```python
from build123d import *

# Parameters (mm, degrees)
SKETCH1_W           = 114.3
SKETCH1_H           = 38.1
BOSS_EXTRUDE1_DEPTH = 25.4
CUT_EXTRUDE1_REACH  = 125.131
SKETCH2_W           = 33.528
SKETCH2_H           = 20.828
CUT_EXTRUDE2_REACH  = 125.131
SKETCH3_R           = 1.778
CUT_EXTRUDE3_REACH  = 125.131
SKETCH4_R           = 1.778
CUT_EXTRUDE4_REACH  = 125.131
SKETCH5_R           = 1.778
SKETCH5_R_2         = 6.35
CUT_EXTRUDE5_REACH  = 125.131
SKETCH6_R           = 1.778
SKETCH6_R_2         = 6.35
CUT_EXTRUDE6_REACH  = 125.131
SKETCH7_R           = 1.778
SKETCH7_R_2         = 6.35
CUT_EXTRUDE7_REACH  = 125.131
SKETCH8_R           = 1.778
SKETCH8_R_2         = 6.35
CUT_EXTRUDE8_REACH  = 125.131
SKETCH9_R           = 1.778
CUT_EXTRUDE9_REACH  = 125.131
SKETCH10_R          = 1.778


with BuildPart() as part:
    # Sketch1 → Boss-Extrude1 (new body)
    with BuildSketch(Plane(origin=(0, 0, 0), x_dir=(1, 0, 0), z_dir=(0, 1, 0))):
        with Locations((-57.15, -19.05)):
            Rectangle(SKETCH1_W, SKETCH1_H)
    extrude(amount=BOSS_EXTRUDE1_DEPTH)

    # Sketch2 → Cut-Extrude1 (cut, up to next)
    with BuildSketch(Plane(origin=(0, 0, 0), x_dir=(0, 0, -1), z_dir=(1, 0, 0)), mode=Mode.PRIVATE) as cut_extrude1_sk1:
        with Locations((-19.05, 12.7)):
            Rectangle(SKETCH2_W, SKETCH2_H)
    cut_extrude1_tool1 = extrude(cut_extrude1_sk1.sketch, amount=-CUT_EXTRUDE1_REACH, mode=Mode.PRIVATE) & part.part
    add(cut_extrude1_tool1.solids().sort_by_distance((0, 12.7, 19.05))[0], mode=Mode.SUBTRACT)

    # Sketch3 → Cut-Extrude2 (cut, up to next)
    with BuildSketch(Plane.XY.offset(38.1), mode=Mode.PRIVATE) as cut_extrude2_sk1:
        with Locations((-2.54, 12.7)):
            Circle(SKETCH3_R)
    cut_extrude2_tool1 = extrude(cut_extrude2_sk1.sketch, amount=-CUT_EXTRUDE2_REACH, mode=Mode.PRIVATE) & part.part
    add(cut_extrude2_tool1.solids().sort_by_distance((-2.54, 12.7, 38.1))[0], mode=Mode.SUBTRACT)

    # Sketch4 → Cut-Extrude3 (cut, up to next)
    with BuildSketch(Plane(origin=(0, 0, 0), x_dir=(-1, 0, 0), z_dir=(0, 0, -1)), mode=Mode.PRIVATE) as cut_extrude3_sk1:
        with Locations(Location((2.54, 12.7, 0), (0, 0, 180))):
            Circle(SKETCH4_R)
    cut_extrude3_tool1 = extrude(cut_extrude3_sk1.sketch, amount=-CUT_EXTRUDE3_REACH, mode=Mode.PRIVATE) & part.part
    add(cut_extrude3_tool1.solids().sort_by_distance((-2.54, 12.7, 0))[0], mode=Mode.SUBTRACT)

    # Sketch5 → Cut-Extrude4 (cut, up to next)
    with BuildSketch(Plane.XY.offset(38.1), mode=Mode.PRIVATE) as cut_extrude4_sk1:
        with Locations((-111.76, 12.7)):
            Circle(SKETCH5_R)
    cut_extrude4_tool1 = extrude(cut_extrude4_sk1.sketch, amount=-CUT_EXTRUDE4_REACH, mode=Mode.PRIVATE) & part.part
    # Sketch5 → Cut-Extrude4 (cut, up to next)
    with BuildSketch(Plane.XY.offset(38.1), mode=Mode.PRIVATE) as cut_extrude4_sk2:
        with Locations((-88.9, 12.7)):
            Circle(SKETCH5_R_2)
    cut_extrude4_tool2 = extrude(cut_extrude4_sk2.sketch, amount=-CUT_EXTRUDE4_REACH, mode=Mode.PRIVATE) & part.part
    # Sketch5 → Cut-Extrude4 (cut, up to next)
    with BuildSketch(Plane.XY.offset(38.1), mode=Mode.PRIVATE) as cut_extrude4_sk3:
        with Locations((-95.814797213, 19.614797213)):
            Circle(SKETCH5_R)
    cut_extrude4_tool3 = extrude(cut_extrude4_sk3.sketch, amount=-CUT_EXTRUDE4_REACH, mode=Mode.PRIVATE) & part.part
    # Sketch5 → Cut-Extrude4 (cut, up to next)
    with BuildSketch(Plane.XY.offset(38.1), mode=Mode.PRIVATE) as cut_extrude4_sk4:
        with Locations((-81.985202787, 19.614797213)):
            Circle(SKETCH5_R)
    cut_extrude4_tool4 = extrude(cut_extrude4_sk4.sketch, amount=-CUT_EXTRUDE4_REACH, mode=Mode.PRIVATE) & part.part
    # Sketch5 → Cut-Extrude4 (cut, up to next)
    with BuildSketch(Plane.XY.offset(38.1), mode=Mode.PRIVATE) as cut_extrude4_sk5:
        with Locations((-95.814797213, 5.785202787)):
            Circle(SKETCH5_R)
    cut_extrude4_tool5 = extrude(cut_extrude4_sk5.sketch, amount=-CUT_EXTRUDE4_REACH, mode=Mode.PRIVATE) & part.part
    # Sketch5 → Cut-Extrude4 (cut, up to next)
    with BuildSketch(Plane.XY.offset(38.1), mode=Mode.PRIVATE) as cut_extrude4_sk6:
        with Locations((-81.985202787, 5.785202787)):
            Circle(SKETCH5_R)
    cut_extrude4_tool6 = extrude(cut_extrude4_sk6.sketch, amount=-CUT_EXTRUDE4_REACH, mode=Mode.PRIVATE) & part.part
    add(cut_extrude4_tool1.solids().sort_by_distance((-111.76, 12.7, 38.1))[0], mode=Mode.SUBTRACT)
    add(cut_extrude4_tool2.solids().sort_by_distance((-88.9, 12.7, 38.1))[0], mode=Mode.SUBTRACT)
    add(cut_extrude4_tool3.solids().sort_by_distance((-95.814797, 19.614797, 38.1))[0], mode=Mode.SUBTRACT)
    add(cut_extrude4_tool4.solids().sort_by_distance((-81.985203, 19.614797, 38.1))[0], mode=Mode.SUBTRACT)
    add(cut_extrude4_tool5.solids().sort_by_distance((-95.814797, 5.785203, 38.1))[0], mode=Mode.SUBTRACT)
    add(cut_extrude4_tool6.solids().sort_by_distance((-81.985203, 5.785203, 38.1))[0], mode=Mode.SUBTRACT)

    # Sketch6 → Cut-Extrude5 (cut, up to next)
    with BuildSketch(Plane(origin=(0, 0, 0), x_dir=(-1, 0, 0), z_dir=(0, 0, -1)), mode=Mode.PRIVATE) as cut_extrude5_sk1:
        with Locations(Location((111.76, 12.7, 0), (0, 0, 180))):
            Circle(SKETCH6_R)
    cut_extrude5_tool1 = extrude(cut_extrude5_sk1.sketch, amount=-CUT_EXTRUDE5_REACH, mode=Mode.PRIVATE) & part.part
    # Sketch6 → Cut-Extrude5 (cut, up to next)
    with BuildSketch(Plane(origin=(0, 0, 0), x_dir=(-1, 0, 0), z_dir=(0, 0, -1)), mode=Mode.PRIVATE) as cut_extrude5_sk2:
        with Locations(Location((88.9, 12.7, 0), (0, 0, 180))):
            Circle(SKETCH6_R_2)
    cut_extrude5_tool2 = extrude(cut_extrude5_sk2.sketch, amount=-CUT_EXTRUDE5_REACH, mode=Mode.PRIVATE) & part.part
    # Sketch6 → Cut-Extrude5 (cut, up to next)
    with BuildSketch(Plane(origin=(0, 0, 0), x_dir=(-1, 0, 0), z_dir=(0, 0, -1)), mode=Mode.PRIVATE) as cut_extrude5_sk3:
        with Locations(Location((81.985202787, 19.614797213, 0), (0, 0, 180))):
            Circle(SKETCH6_R)
    cut_extrude5_tool3 = extrude(cut_extrude5_sk3.sketch, amount=-CUT_EXTRUDE5_REACH, mode=Mode.PRIVATE) & part.part
    # Sketch6 → Cut-Extrude5 (cut, up to next)
    with BuildSketch(Plane(origin=(0, 0, 0), x_dir=(-1, 0, 0), z_dir=(0, 0, -1)), mode=Mode.PRIVATE) as cut_extrude5_sk4:
        with Locations(Location((95.814797213, 19.614797213, 0), (0, 0, 180))):
            Circle(SKETCH6_R)
    cut_extrude5_tool4 = extrude(cut_extrude5_sk4.sketch, amount=-CUT_EXTRUDE5_REACH, mode=Mode.PRIVATE) & part.part
    # Sketch6 → Cut-Extrude5 (cut, up to next)
    with BuildSketch(Plane(origin=(0, 0, 0), x_dir=(-1, 0, 0), z_dir=(0, 0, -1)), mode=Mode.PRIVATE) as cut_extrude5_sk5:
        with Locations(Location((95.814797213, 5.785202787, 0), (0, 0, 180))):
            Circle(SKETCH6_R)
    cut_extrude5_tool5 = extrude(cut_extrude5_sk5.sketch, amount=-CUT_EXTRUDE5_REACH, mode=Mode.PRIVATE) & part.part
    # Sketch6 → Cut-Extrude5 (cut, up to next)
    with BuildSketch(Plane(origin=(0, 0, 0), x_dir=(-1, 0, 0), z_dir=(0, 0, -1)), mode=Mode.PRIVATE) as cut_extrude5_sk6:
        with Locations(Location((81.985202787, 5.785202787, 0), (0, 0, 180))):
            Circle(SKETCH6_R)
    cut_extrude5_tool6 = extrude(cut_extrude5_sk6.sketch, amount=-CUT_EXTRUDE5_REACH, mode=Mode.PRIVATE) & part.part
    add(cut_extrude5_tool1.solids().sort_by_distance((-111.76, 12.7, 0))[0], mode=Mode.SUBTRACT)
    add(cut_extrude5_tool2.solids().sort_by_distance((-88.9, 12.7, 0))[0], mode=Mode.SUBTRACT)
    add(cut_extrude5_tool3.solids().sort_by_distance((-81.985203, 19.614797, 0))[0], mode=Mode.SUBTRACT)
    add(cut_extrude5_tool4.solids().sort_by_distance((-95.814797, 19.614797, 0))[0], mode=Mode.SUBTRACT)
    add(cut_extrude5_tool5.solids().sort_by_distance((-95.814797, 5.785203, 0))[0], mode=Mode.SUBTRACT)
    add(cut_extrude5_tool6.solids().sort_by_distance((-81.985203, 5.785203, 0))[0], mode=Mode.SUBTRACT)

    # Sketch7 → Cut-Extrude6 (cut, up to next)
    with BuildSketch(Plane(origin=(0, 25.4, 0), x_dir=(1, 0, 0), z_dir=(0, 1, 0)), mode=Mode.PRIVATE) as cut_extrude6_sk1:
        with Locations(Location((-111.76, -19.05, 0), (0, 0, 270))):
            Circle(SKETCH7_R)
    cut_extrude6_tool1 = extrude(cut_extrude6_sk1.sketch, amount=-CUT_EXTRUDE6_REACH, mode=Mode.PRIVATE) & part.part
    # Sketch7 → Cut-Extrude6 (cut, up to next)
    with BuildSketch(Plane(origin=(0, 25.4, 0), x_dir=(1, 0, 0), z_dir=(0, 1, 0)), mode=Mode.PRIVATE) as cut_extrude6_sk2:
        with Locations(Location((-88.9, -19.05, 0), (0, 0, 270))):
            Circle(SKETCH7_R_2)
    cut_extrude6_tool2 = extrude(cut_extrude6_sk2.sketch, amount=-CUT_EXTRUDE6_REACH, mode=Mode.PRIVATE) & part.part
    # Sketch7 → Cut-Extrude6 (cut, up to next)
    with BuildSketch(Plane(origin=(0, 25.4, 0), x_dir=(1, 0, 0), z_dir=(0, 1, 0)), mode=Mode.PRIVATE) as cut_extrude6_sk3:
        Polygon((-61.468, -19.05), (-61.468, -9.017), (-20.574, -9.017), (-20.574, -29.083), (-61.468, -29.083), align=None)
    cut_extrude6_tool3 = extrude(cut_extrude6_sk3.sketch, amount=-CUT_EXTRUDE6_REACH, mode=Mode.PRIVATE) & part.part
    add(cut_extrude6_tool1.solids().sort_by_distance((-111.76, 25.4, 19.05))[0], mode=Mode.SUBTRACT)
    add(cut_extrude6_tool2.solids().sort_by_distance((-88.9, 25.4, 19.05))[0], mode=Mode.SUBTRACT)
    add(cut_extrude6_tool3.solids().sort_by_distance((-41.021, 25.4, 19.05))[0], mode=Mode.SUBTRACT)

    # Sketch8 → Cut-Extrude7 (cut, up to next)
    with BuildSketch(Plane.XZ, mode=Mode.PRIVATE) as cut_extrude7_sk1:
        with Locations(Location((-111.76, 19.05, 0), (0, 0, 90))):
            Circle(SKETCH8_R)
    cut_extrude7_tool1 = extrude(cut_extrude7_sk1.sketch, amount=-CUT_EXTRUDE7_REACH, mode=Mode.PRIVATE) & part.part
    # Sketch8 → Cut-Extrude7 (cut, up to next)
    with BuildSketch(Plane.XZ, mode=Mode.PRIVATE) as cut_extrude7_sk2:
        with Locations(Location((-88.9, 19.05, 0), (0, 0, 90))):
            Circle(SKETCH8_R_2)
    cut_extrude7_tool2 = extrude(cut_extrude7_sk2.sketch, amount=-CUT_EXTRUDE7_REACH, mode=Mode.PRIVATE) & part.part
    # Sketch8 → Cut-Extrude7 (cut, up to next)
    with BuildSketch(Plane.XZ, mode=Mode.PRIVATE) as cut_extrude7_sk3:
        Polygon((-61.468, 19.05), (-61.468, 29.083), (-20.574, 29.083), (-20.574, 9.017), (-61.468, 9.017), align=None)
    cut_extrude7_tool3 = extrude(cut_extrude7_sk3.sketch, amount=-CUT_EXTRUDE7_REACH, mode=Mode.PRIVATE) & part.part
    add(cut_extrude7_tool1.solids().sort_by_distance((-111.76, 0, 19.05))[0], mode=Mode.SUBTRACT)
    add(cut_extrude7_tool2.solids().sort_by_distance((-88.9, 0, 19.05))[0], mode=Mode.SUBTRACT)
    add(cut_extrude7_tool3.solids().sort_by_distance((-41.021, 0, 19.05))[0], mode=Mode.SUBTRACT)

    # Sketch9 → Cut-Extrude8 (cut, up to next)
    with BuildSketch(Plane(origin=(0, 25.4, 0), x_dir=(1, 0, 0), z_dir=(0, 1, 0)), mode=Mode.PRIVATE) as cut_extrude8_sk1:
        with Locations(Location((-2.54, -19.05, 0), (0, 0, 270))):
            Circle(SKETCH9_R)
    cut_extrude8_tool1 = extrude(cut_extrude8_sk1.sketch, amount=-CUT_EXTRUDE8_REACH, mode=Mode.PRIVATE) & part.part
    add(cut_extrude8_tool1.solids().sort_by_distance((-2.54, 25.4, 19.05))[0], mode=Mode.SUBTRACT)

    # Sketch10 → Cut-Extrude9 (cut, up to next)
    with BuildSketch(Plane(origin=(0, 0, 0), x_dir=(-1, 0, 0), z_dir=(0, -1, 0)), mode=Mode.PRIVATE) as cut_extrude9_sk1:
        with Locations(Location((2.54, -19.05, 0), (0, 0, 270))):
            Circle(SKETCH10_R)
    cut_extrude9_tool1 = extrude(cut_extrude9_sk1.sketch, amount=-CUT_EXTRUDE9_REACH, mode=Mode.PRIVATE) & part.part
    add(cut_extrude9_tool1.solids().sort_by_distance((-2.54, 0, 19.05))[0], mode=Mode.SUBTRACT)


solid = part.part
```
The listing builds one solid part. Answer for the finished solid, in the listing's coordinates (mm). A direction names the side the tool comes from. Round coordinates to 2 decimals unless told otherwise and drop trailing zeros. Loops run counter-clockwise (first coordinate to the right, second up) from the corner with the lowest first, then second, coordinate; pieces in that order, holes last.
Q1. Find the intervals of material crossed by line 1 (X direction, y = 1.2, z = 19.05); line 2 (Y direction, x = -81, z = 9.5); line 3 (Z direction, x = -9.5, y = 10.75), in increasing order.
Q2. Section A-A, the plane x = -88.9 is taken. Determine the outline of the cut face in (y, z), then the cut area to 3 significant figures.
Q3. Section D-D, the plane x = -45 is taken. Determine the outline of the cut face in (y, z), then the cut area to 3 significant figures.
Q4. Section B-B, the plane z = 11.5 is taken. Determine the outline of the cut face in (x, y).
Q5. Which of the six approach directions +Z, -Z, +X, -X, +Y, -Y give full straight-line access (tool end or side, diameter ignored) to faces 1 (the face through (0, 1, 19)), 2 (the face through (-41, 1, 29.083))?
Q6. Section C-C, the plane y = 12.7 is taken. Count the separate pieces of the cut face and the enclosed holes in it, then the cut area to 3 significant figures.
Q7. For a pull along Z with two mould halves and no side action, classify faces 3 (the face through (-69, 23.114, 19)), 4 (the face through (-97.59, 19.54, 1.13)), 5 (the face through (-58, 13, 0)) as released by +Z, released by -Z, zero draft, split by the parting line, or undercut.
Q8. Given pin 1 Ø10 at (x, y) = (-88.9, 12.7) entering from -Z, flat-ended and moving along its own axis, determine where the tip first touches the part or whether it passes through.
Completed:
1. line 1: x = -114.3 to -113.54, -109.98 to -95.25, -82.55 to -61.47, -20.57 to -4.32, -0.76 to 0
1. line 2: y = 0 to 2.29, 23.11 to 25.4
1. line 3: z = 0 to 2.29, 35.81 to 38.1
2. outline: (0, 0) - (6.35, 0) - (6.35, 2.29) - (2.29, 2.29) - (2.29, 12.7) - (0, 12.7) - close; (0, 25.4) - (2.29, 25.4) - (2.29, 35.81) - (6.35, 35.81) - (6.35, 38.1) - (0, 38.1) - close; (19.05, 0) - (25.4, 0) - (25.4, 12.7) - (23.11, 12.7) - (23.11, 2.29) - (19.05, 2.29) - close; (19.05, 35.81) - (23.11, 35.81) - (23.11, 25.4) - (25.4, 25.4) - (25.4, 38.1) - (19.05, 38.1) - close
2. area: 153 mm2
3. outline: (0, 0) - (25.4, 0) - (25.4, 9.02) - (23.11, 9.02) - (23.11, 2.29) - (2.29, 2.29) - (2.29, 9.02) - (0, 9.02) - close; (0, 29.08) - (2.29, 29.08) - (2.29, 35.81) - (23.11, 35.81) - (23.11, 29.08) - (25.4, 29.08) - (25.4, 38.1) - (0, 38.1) - close
3. area: 178 mm2
4. outline: (-114.3, 0) - (-61.47, 0) - (-61.47, 2.29) - (-114.3, 2.29) - close; (-114.3, 23.11) - (-61.47, 23.11) - (-61.47, 25.4) - (-114.3, 25.4) - close; (-20.57, 0) - (0, 0) - (0, 2.29) - (-20.57, 2.29) - close; (-20.57, 23.11) - (0, 23.11) - (0, 25.4) - (-20.57, 25.4) - close
5. face 1: +Z, -Z, +X, +Y, -Y
5. face 2: +Y, -Y
6. separate pieces: 8
6. enclosed holes: 0
6. area: 432 mm2
7. face 3: undercut
7. face 4: zero draft
7. face 5: released by -Z
8. pin 1: passes through
